Verification items for this drawing (mm, ordinates from the low corner). A direction names the side the tool comes from. Round coordinates to 2 decimals unless told otherwise and drop trailing zeros. Order: outer loops, then holes, each group sorted by start corner. A loop starts at its lowest first (then second) coordinate and runs counter-clockwise, first axis right, second up. Notation, with made-up numbers: (7.5, 28.25) - (56.5, 28.25) arc R28 ccw to (56.5, 63.25) - close; hole circle Ø9 at (42, 24.5). An arc over 180 degrees is marked (long way). Use a Markdown table: item, result. Add a question column.
(1) Section check A-A on x = 66. Record the boundary of the cut face in (y, z).
(2) Section check D-D on z = 88. Record the boundary of the cut face in (x, y).
(3) Mould release check, pull along Y, two halves, no side actions. Record for the marked faces 4, 5 and 6: released by +Y, released by -Y, zero draft, split by the parting line, or undercut.
(4) Access from +Z, -Z, +X, -X, +Y, -Y to the whole of each face (thin tool, end or side, straight path). Record for the marked faces 1, 2 and 3.
(5) Thickness scan on line 1 along Z through (x, y) = (60, 0.8); line 2 along Y through (x, z) = (65, 93.5); line 3 along X through (y, z) = (25, 66). Record the ranges inside material, lowest first. Write a range as [from, to].
(6) Gauge pin test, flat ends, axial feed: P1, Ø4, axis at x = 25, z = 75, coming from the +Y side; P2, Ø0.6, axis at y = 30.5, z = 37.5, coming from the +X side; P3, Ø8.5, axis at x = 39.5, y = 14, coming from the +Z side; P4, Ø1.5, axis at x = 81.5, y = 8, coming from the -Z side. Record the tip position at first contact, or that the pin passes through.
(7) Section check B-B on z = 29. Record the boundary of the cut face in (x, y), then the cut area to 3 significant figures.
(8) Section check C-C on y = 8. Record the boundary of the cut face in (x, z), then the cut area to 3 significant figures.
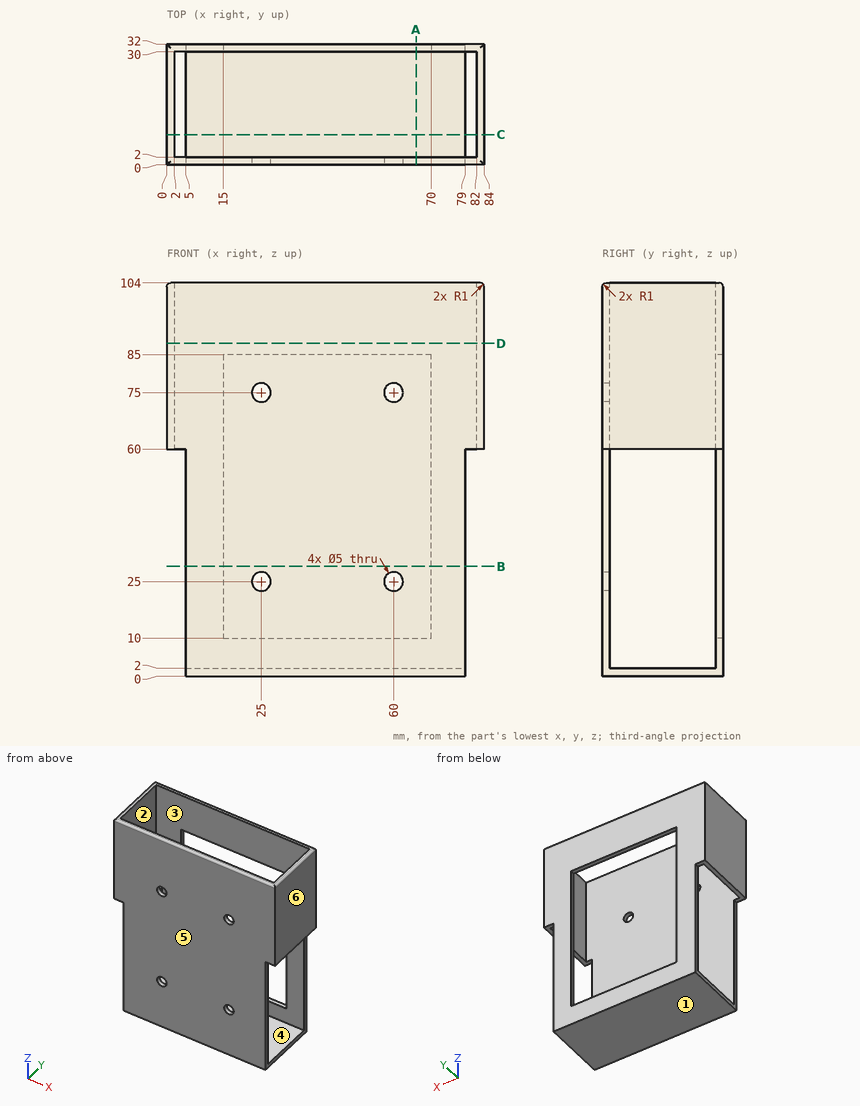
Check sheet entries:
| question | item | result |
|---|---|---|
| 1 | outline | (0, 0) - (32, 0) - (32, 10) - (30, 10) - (30, 2) - (2, 2) - (2, 104) - (1, 104) arc R1 ccw to (0, 103) - close; (30, 85) - (32, 85) - (32, 103) arc R1 ccw to (31, 104) - (30, 104) - close |
| 2 | outline | (0, 0) - (84, 0) - (84, 32) - (0, 32) - close; hole (2, 2) - (82, 2) - (82, 30) - (2, 30) - close |
| 3 | face 4 | undercut |
| 3 | face 5 | released by -Y |
| 3 | face 6 | zero draft |
| 4 | face 1 | -Z, +X, -X, +Y, -Y |
| 4 | face 2 | +Z, -Z |
| 4 | face 3 | +Z |
| 5 | line 1 | z = [0, 22.5], [27.5, 72.5], [77.5, 103.98] |
| 5 | line 2 | y = [0, 2], [30, 32] |
| 5 | line 3 | x = [0, 2], [82, 84] |
| 6 | P1 | passes through |
| 6 | P2 | stops at x = 79 |
| 6 | P3 | stops at z = 2 |
| 6 | P4 | stops at z = 60 |
| 7 | outline | (5, 0) - (79, 0) - (79, 2) - (5, 2) - close; (5, 30) - (15, 30) - (15, 32) - (5, 32) - close; (70, 30) - (79, 30) - (79, 32) - (70, 32) - close |
| 7 | area | 186 mm2 |
| 8 | outline | (0, 60) - (2, 60) - (2, 104) - (1, 104) arc R1 ccw to (0, 103) - close; (5, 0) - (79, 0) - (79, 2) - (5, 2) - close; (82, 60) - (84, 60) - (84, 103) arc R1 ccw to (83, 104) - (82, 104) - close |
| 8 | area | 324 mm2 |
